from build123d import *

# Parameters (mm, degrees)
SKETCH1_W           = 45
SKETCH1_H           = 160
BOSS_EXTRUDE1_DEPTH = 5.08
SKETCH2_W           = 5.08
SKETCH2_H           = 10
BOSS_EXTRUDE2_DEPTH = 5.08
SKETCH3_W           = 35
SKETCH3_H           = 13
SKETCH3_H_2         = 29.5
SKETCH3_H_3         = 37.5
SKETCH3_H_4         = 10
SKETCH3_H_5         = 40
CUT_EXTRUDE1_DEPTH  = 6.08
BOSS_EXTRUDE3_DEPTH = 5.08
FILLET1_R           = 0.5


with BuildPart() as part:
    # Sketch1 → Boss-Extrude1 (new body)
    with BuildSketch(Plane(origin=(0, 0, 0), x_dir=(1, 0, 0), z_dir=(0, 1, 0))):
        Rectangle(SKETCH1_W, SKETCH1_H)
    extrude(amount=BOSS_EXTRUDE1_DEPTH)

    # Sketch2 → Boss-Extrude2 (add)
    with BuildSketch(Plane(origin=(0, 5.08, 0), x_dir=(1, 0, 0), z_dir=(0, 1, 0))):
        with Locations((25.04, 25)):
            Rectangle(SKETCH2_W, SKETCH2_H)
        with Locations((25.04, 75)):
            Rectangle(SKETCH2_W, SKETCH2_H)
        with Locations((25.04, -25)):
            Rectangle(SKETCH2_W, SKETCH2_H)
        with Locations((25.04, -75)):
            Rectangle(SKETCH2_W, SKETCH2_H)
    boss_extrude2 = extrude(amount=-BOSS_EXTRUDE2_DEPTH)

    # Mirror1: Boss-Extrude2 across plane
    add(boss_extrude2.mirror(Plane(origin=(0, 0, 0), x_dir=(0, 0, 1), z_dir=(1, 0, 0))))

    # Sketch3 → Cut-Extrude1 (cut, through all)
    with BuildSketch(Plane(origin=(0, 5.08, 0), x_dir=(1, 0, 0), z_dir=(0, 1, 0))):
        with Locations((0, 68.5)):
            Rectangle(SKETCH3_W, SKETCH3_H)
        with Locations((0, 42.25)):
            Rectangle(SKETCH3_W, SKETCH3_H_2)
        with Locations((0, 3.75)):
            Rectangle(SKETCH3_W, SKETCH3_H_3)
        with Locations((0, -25)):
            Rectangle(SKETCH3_W, SKETCH3_H_4)
        with Locations((0, -55)):
            Rectangle(SKETCH3_W, SKETCH3_H_5)
    extrude(amount=-CUT_EXTRUDE1_DEPTH, mode=Mode.SUBTRACT)

    # Sketch4 → Boss-Extrude3 (add)
    with BuildSketch(Plane(origin=(0, 5.08, 0), x_dir=(1, 0, 0), z_dir=(0, 1, 0))):
        Polygon((-17.5, -40.315072906), (-4.650688793, -55), (-17.5, -69.684927094), (-17.5, -75), (-12.849311207, -75), (0, -60.315072906), (12.849311207, -75), (17.5, -75), (17.5, -69.684927094), (4.650688793, -55), (17.5, -40.315072906), (17.5, -35), (12.849311207, -35), (0, -49.684927094), (-12.849311207, -35), (-17.5, -35), align=None)
        Polygon((-12.712400277, 22.5), (0, 8.879571132), (12.712400277, 22.5), (17.5, 22.5), (17.5, 17.370428868), (4.787599723, 3.75), (17.5, -9.870428868), (17.5, -15), (12.712400277, -15), (0, -1.379571132), (-12.712400277, -15), (-17.5, -15), (-17.5, -9.870428868), (-4.787599723, 3.75), (-17.5, 17.370428868), (-17.5, 22.5), align=None)
        Polygon((-17.5, 52.422609914), (-5.430801797, 42.25), (-17.5, 32.077390086), (-17.5, 27.5), (-12.069198203, 27.5), (0, 37.672609914), (12.069198203, 27.5), (17.5, 27.5), (17.5, 32.077390086), (5.430801797, 42.25), (17.5, 52.422609914), (17.5, 57), (12.069198203, 57), (0, 46.827390086), (-12.069198203, 57), (-17.5, 57), align=None)
    extrude(amount=-BOSS_EXTRUDE3_DEPTH)

    # Fillet1
    fillet1_edges = [part.edges().sort_by_distance(p)[0] for p in [
        (-17.5, 2.54, -62),
        (-17.5, 2.54, -75),
        (17.5, 2.54, -75),
        (17.5, 2.54, -62),
        (-17.5, 2.54, 30),
        (-17.5, 2.54, 20),
        (17.5, 2.54, 20),
        (17.5, 2.54, 30),
        (-12.849311207, 2.54, 75),
        (-17.5, 2.54, 69.684927094),
        (-4.650688793, 2.54, 55),
        (-17.5, 2.54, 40.315072906),
        (-12.849311207, 2.54, 35),
        (0, 2.54, 49.684927094),
        (12.849311207, 2.54, 35),
        (17.5, 2.54, 40.315072906),
        (4.650688793, 2.54, 55),
        (17.5, 2.54, 69.684927094),
        (12.849311207, 2.54, 75),
        (0, 2.54, 60.315072906),
        (-17.5, 2.54, 9.870428868),
        (-4.787599723, 2.54, -3.75),
        (-17.5, 2.54, -17.370428868),
        (-12.712400277, 2.54, -22.5),
        (0, 2.54, -8.879571132),
        (12.712400277, 2.54, -22.5),
        (17.5, 2.54, -17.370428868),
        (4.787599723, 2.54, -3.75),
        (17.5, 2.54, 9.870428868),
        (12.712400277, 2.54, 15),
        (0, 2.54, 1.379571132),
        (-12.712400277, 2.54, 15),
        (-12.069198203, 2.54, -27.5),
        (-17.5, 2.54, -32.077390086),
        (-5.430801797, 2.54, -42.25),
        (-17.5, 2.54, -52.422609914),
        (-12.069198203, 2.54, -57),
        (0, 2.54, -46.827390086),
        (12.069198203, 2.54, -57),
        (17.5, 2.54, -52.422609914),
        (5.430801797, 2.54, -42.25),
        (17.5, 2.54, -32.077390086),
        (12.069198203, 2.54, -27.5),
        (0, 2.54, -37.672609914),
    ]]
    fillet(fillet1_edges, radius=FILLET1_R)


solid = part.part
Here's how the part is built. I have some questions about the finished solid (model axes, mm). A direction names the side the tool comes from. Give positions to 0.01 mm unless a question says otherwise; leave off trailing zeros. Order: outer loops, then holes, each group sorted by start corner. A loop starts at its lowest first (then second) coordinate and runs counter-clockwise, first axis right, second up. Notation, with made-up numbers: M 16,-7 L 66,-7 A21 ccw 66,29 Z; hole C 4.25,77.25 d7. An arc over 180 degrees is marked long. Answer as a JSON object with one key per item and string values. Group by question number.
1) Suppose I cut it at C-C, the plane y = 1.25. Count the separate pieces of the cut face and the enclosed holes in it, plus the area to 3 significant figures.
2) Please list where these lines run through material, in increasing order: L1, parallel to Z at x = -23, y = 3.3; L2, parallel to X at y = 3.2, z = 44.5; L3, parallel to X at y = 3, z = 25.5. Write a range as [from, to].
3) Suppose I cut it at D-D, the plane z = -13.5. Write out the boundary of the cut face in (x, y).
4) I'm going to push flat-ended pins straight in: pin 1 Ø1 at (y, z) = (0.5, 56) entering from +X; pin 2 Ø1.5 at (y, z) = (3.5, -7.5) entering from -X. Where does each tip first touch, or does it pass through?
5) Suppose I cut it at B-B, the plane z = 27. Write out the boundary of the cut face in (x, y), plus the area to 3 significant figures.
6) Suppose I cut it at A-A, the plane z = 47. Write out the boundary of the cut face in (x, y), plus the area to 3 significant figures.
7) We'd pull the mould along X, two halves only. Please class faces 1 (the flat face through (-25, 3, 70)), 2 (the flat face through (0, 3, -27.5)), 3 (the flat face through (-27.58, 3, 75)): pulls with the +X half, pulls with the -X half, needs draft (parallel to the pull), parting line crosses it, or undercut.
8) On a 3-axis mill with a long thin cutter (end or side, diameter ignored), from which of +Z, -Z, +X, -X, +Y, -Y can I reach the whole of each face in a straight line? I mean faces 4 (the flat face through (25, 3, 20)), 5 (the flat face through (10.95, 2.58, -10.35)), 6 (the flat face through (-27.58, 3, -25)). Say none if no direction works.
Results found:
{
 "1": {"separate pieces": "1", "enclosed holes": "14", "area": "4,870 mm²"},
 "2": {"L1": "[-80, -70], [-30, -20], [20, 30], [70, 80]", "L2": "[-22.5, -17.5], [-13.84, -4.54], [4.54, 13.84], [17.5, 22.5]", "L3": "[-27.58, -17.5], [17.5, 27.58]"},
 "3": {"outline": "M -22.5,0 L -17.5,0 L -17.5,5.08 L -22.5,5.08 Z; M -13.89,0 L -4.31,0 L -4.31,5.08 L -13.89,5.08 Z; M 4.31,0 L 13.89,0 L 13.89,5.08 L 4.31,5.08 Z; M 17.5,0 L 22.5,0 L 22.5,5.08 L 17.5,5.08 Z"},
 "4": {"pin 1": "x = 22.5", "pin 2": "x = -22.5"},
 "5": {"outline": "M -27.58,0 L -17.5,0 L -17.5,5.08 L -27.58,5.08 Z; M 17.5,0 L 27.58,0 L 27.58,5.08 L 17.5,5.08 Z", "area": "102 mm²"},
 "6": {"outline": "M -22.5,0 L -17.5,0 L -17.5,5.08 L -22.5,5.08 Z; M -11.65,0 L -2.35,0 L -2.35,5.08 L -11.65,5.08 Z; M 2.35,0 L 11.65,0 L 11.65,5.08 L 2.35,5.08 Z; M 17.5,0 L 22.5,0 L 22.5,5.08 L 17.5,5.08 Z", "area": "145 mm²"},
 "7": {"face 1": "needs draft", "face 2": "undercut", "face 3": "pulls with the -X half"},
 "8": {"face 4": "+X, +Y, -Y", "face 5": "+Y, -Y", "face 6": "+Z, -Z, -X, +Y, -Y"}
}
